Geometry check sheet. Reference: the model listing, model coordinates, mm. A direction names the side the tool comes from. Coordinates: 2 decimals unless noted, no trailing zeros. Write each loop counter-clockwise with the first axis right and the second up, starting at its lowest first coordinate (ties: lowest second). Pieces come first, ordered by that corner, then holes. Notation, with made-up numbers: (-23.75, -20.5) -> (1.25, -20.5) arc R17 cw to (1.25, -15.5) -> close; hole circle Ø1 at (66.25, 2). An arc over 180 degrees is marked (long way). One line per question, with ' | ' between items.
```python
from build123d import *

# Parameters (mm, degrees)
CUT_EXTRUDE1_REACH = 191.239
SKETCH2_R          = 3.175


with BuildPart() as part:
    # Sketch1 → Revolve1 (revolve)
    with BuildSketch(Plane.XY):
        with BuildLine():
            Line((0, 0), (-78.74, 0))
            Line((-78.74, 0), (-85.09, 0))
            Line((-85.09, 0), (-57.15, 152.4))
            Line((-57.15, 152.4), (-50.8, 152.4))
            Line((-50.8, 152.4), (-50.8, 8.89))
            ThreePointArc((-50.8, 8.89), (-50.056051224, 7.093948776), (-48.26, 6.35))
            Line((-48.26, 6.35), (0, 6.35))
            Line((0, 6.35), (0, 0))
        make_face()
        with BuildLine():
            Line((-57.15, 8.89), (-57.15, 117.763636364))
            Line((-57.15, 117.763636364), (-77.026193989, 9.348032787))
            ThreePointArc((-77.026193989, 9.348032787), (-76.479115384, 7.263931625), (-74.527833333, 6.35))
            Line((-74.527833333, 6.35), (-59.69, 6.35))
            ThreePointArc((-59.69, 6.35), (-57.893948776, 7.093948776), (-57.15, 8.89))
        make_face(mode=Mode.SUBTRACT)
    revolve(axis=Axis((0, 152.4, 0), (0, -1, 0)))

    # Sketch2 → Cut-Extrude1 (cut, up to next)
    with BuildSketch(Plane(origin=(0, 6.35, 0), x_dir=(1, 0, 0), z_dir=(0, 1, 0)), mode=Mode.PRIVATE) as cut_extrude1_sk1:
        with Locations(Location((0, 0, 0), (0, 0, 180))):
            Circle(SKETCH2_R)
    cut_extrude1_tool1 = extrude(cut_extrude1_sk1.sketch, amount=-CUT_EXTRUDE1_REACH, mode=Mode.PRIVATE) & part.part
    # Sketch2 → Cut-Extrude1 (cut, up to next)
    with BuildSketch(Plane(origin=(0, 6.35, 0), x_dir=(1, 0, 0), z_dir=(0, 1, 0)), mode=Mode.PRIVATE) as cut_extrude1_sk2:
        with Locations(Location((25.4, 0, 0), (0, 0, 180))):
            Circle(SKETCH2_R)
    cut_extrude1_tool2 = extrude(cut_extrude1_sk2.sketch, amount=-CUT_EXTRUDE1_REACH, mode=Mode.PRIVATE) & part.part
    # Sketch2 → Cut-Extrude1 (cut, up to next)
    with BuildSketch(Plane(origin=(0, 6.35, 0), x_dir=(1, 0, 0), z_dir=(0, 1, 0)), mode=Mode.PRIVATE) as cut_extrude1_sk3:
        with Locations(Location((-25.4, 0, 0), (0, 0, 180))):
            Circle(SKETCH2_R)
    cut_extrude1_tool3 = extrude(cut_extrude1_sk3.sketch, amount=-CUT_EXTRUDE1_REACH, mode=Mode.PRIVATE) & part.part
    add(cut_extrude1_tool1.solids().sort_by_distance((0, 6.35, 0))[0], mode=Mode.SUBTRACT)
    add(cut_extrude1_tool2.solids().sort_by_distance((25.4, 6.35, 0))[0], mode=Mode.SUBTRACT)
    add(cut_extrude1_tool3.solids().sort_by_distance((-25.4, 6.35, 0))[0], mode=Mode.SUBTRACT)


solid = part.part
```
(1) Cross-section at A-A (x = 0). Record the cut outline in (y, z) (3 decimals).
Answers below:
outline: (0, -85.09) -> (152.4, -57.15) -> (152.4, -50.8) -> (8.89, -50.8) arc R2.54 cw to (6.35, -48.26) -> (6.35, -3.175) -> (0, -3.175) -> close; (0, 3.175) -> (6.35, 3.175) -> (6.35, 48.26) arc R2.54 cw to (8.89, 50.8) -> (152.4, 50.8) -> (152.4, 57.15) -> (0, 85.09) -> close; hole (6.35, -74.528) arc R2.54 ccw to (9.348, -77.026) -> (117.764, -57.15) -> (8.89, -57.15) arc R2.54 ccw to (6.35, -59.69) -> close; hole (6.35, 59.69) arc R2.54 ccw to (8.89, 57.15) -> (117.764, 57.15) -> (9.348, 77.026) arc R2.54 ccw to (6.35, 74.528) -> close
(2) Cross-section at B-B (z = 0). Count the separate pieces of the cut face and the enclosed holes in it, plus the area to 3 significant figures.
Answers below:
separate pieces: 4 | enclosed holes: 2 | area: 4,450 mm²
(3) Draft check along X on faces 1 (the face through (38, 152.4, 34)), 2 (the face through (14.702, 94.2, 66.207)), 3 (the face through (14.095, 74.843, 63.473)). Enter one of: pulls with the +X half, pulls with the -X half, needs draft (parallel to the pull), parting line crosses it, or undercut.
Answers below:
face 1: needs draft | face 2: parting line crosses it | face 3: undercut
(4) Cross-section at C-C (y = 51). Record the cut outline in (x, z), plus the area to 3 significant figures.
Answers below:
outline: circle Ø151.48 at (0, 0); circle Ø114.3 at (0, 0); hole circle Ø138.78 at (0, 0); hole circle Ø101.6 at (0, 0) | area: 5,050 mm²
(5) Tool access check on faces 4 (the face through (1, 6.35, 10)), 5 (the face through (57.095, 64.089, -2.513)), 6 (the face through (-1, 0, 18)). Record the directions out of +Z, -Z, +X, -X, +Y, -Y that give a thin tool (end or side, any length) a straight path to the whole face; none if there is none.
Answers below:
face 4: +Y | face 5: none | face 6: +Z, -Z, +X, -X, -Y
(6) Material ranges on line 1 (X direction, y = 52, z = -33); line 2 (Z direction, x = -29.5, y = 103); line 3 (Z direction, x = -13, y = 25.5), recorded low to high.
Answers below:
line 1: x = -67.97 to -60.83, -46.66 to -38.62, 38.62 to 46.66, 60.83 to 67.97 | line 2: z = -59.27 to -52.08, -48.95 to -41.36, 41.36 to 48.95, 52.08 to 59.27 | line 3: z = -79.36 to -72.92, -55.65 to -49.11, 49.11 to 55.65, 72.92 to 79.36
(7) Cross-section at D-D (y = 27). Record the cut outline in (x, z).
Answers below:
outline: circle Ø160.28 at (0, 0); circle Ø114.3 at (0, 0); hole circle Ø147.58 at (0, 0); hole circle Ø101.6 at (0, 0)
(8) Depth check by flat-ended pin: P1, Ø6, axis at x = -32, z = -39, coming from the +Y side; P2, Ø2, axis at y = 40.5, z = 62.5, coming from the +X side; P3, Ø5, axis at x = -2.5, y = 18, coming from the +Z side; P4, Ø12, axis at x = -32.5, y = 94.5, coming from the +Z side. Enter the tip coordinate at first touch or a pass-through.
Answers below:
P1: stops at y = 152.4 | P2: stops at x = 47.46 | P3: stops at z = 82.22 | P4: stops at z = 62.63
